from build123d import *

# Parameters (mm, degrees)
BOSS_EXTRUDE1_DEPTH                                  = 300
SKETCH2_R                                            = 30
CUT_EXTRUDE1_DEPTH                                   = 319.198051534
SKETCH3_W                                            = 40
SKETCH3_H                                            = 56
CUT_EXTRUDE2_DEPTH                                   = 10
SKETCH4_W                                            = 40
SKETCH4_H                                            = 49
CUT_EXTRUDE3_DEPTH                                   = 10
FILLET1_R                                            = 3
CSK_FOR_M10_COUNTERSUNK_FLAT_HEAD_SCREW1_D           = 11
CSK_FOR_M10_COUNTERSUNK_FLAT_HEAD_SCREW1_DEPTH       = 20.003
CSK_FOR_M10_COUNTERSUNK_FLAT_HEAD_SCREW1_CSINK_D     = 20
CSK_FOR_M10_COUNTERSUNK_FLAT_HEAD_SCREW1_CSINK_ANGLE = 90
CSK_FOR_M10_COUNTERSUNK_FLAT_HEAD_SCREW1_TIP         = 3.304733405
BOSS_EXTRUDE2_START                                  = -6.35
SKETCH7_R                                            = 30
SKETCH7_R_2                                          = 22.5
BOSS_EXTRUDE2_DEPTH                                  = 6.35
M6X1_0_TAPPED_HOLE1_D                                = 5
M6X1_0_TAPPED_HOLE1_DEPTH                            = 15
M6X1_0_TAPPED_HOLE1_CSINK_D                          = 6.05
M6X1_0_TAPPED_HOLE1_CSINK_ANGLE                      = 90
M6X1_0_TAPPED_HOLE1_TIP                              = 1.502151548


with BuildPart() as part:
    # Sketch1 → Boss-Extrude1 (new body)
    with BuildSketch(Plane.XY):
        Polygon((0, -37.5), (0, 37.5), (75, 37.5), (75, 31.15), (6.35, 31.15), (6.35, -31.15), (75, -31.15), (75, -37.5), align=None)
    extrude(amount=BOSS_EXTRUDE1_DEPTH)

    # Sketch2 → Cut-Extrude1 (cut, through all)
    with BuildSketch(Plane(origin=(0, 37.5, 0), x_dir=(1, 0, 0), z_dir=(0, 1, 0))):
        with Locations(Location((40, -150, 0), (0, 0, 270))):
            Circle(SKETCH2_R)
    extrude(amount=-CUT_EXTRUDE1_DEPTH, mode=Mode.SUBTRACT)

    # Sketch3 → Cut-Extrude2 (cut)
    with BuildSketch(Plane.XZ.offset(37.5)):
        with Locations((40, 63)):
            Rectangle(SKETCH3_W, SKETCH3_H)
    extrude(amount=-CUT_EXTRUDE2_DEPTH, mode=Mode.SUBTRACT)

    # Sketch4 → Cut-Extrude3 (cut)
    with BuildSketch(Plane(origin=(0, 37.5, 0), x_dir=(1, 0, 0), z_dir=(0, 1, 0))):
        with Locations((40, -82.5)):
            Rectangle(SKETCH4_W, SKETCH4_H)
    extrude(amount=-CUT_EXTRUDE3_DEPTH, mode=Mode.SUBTRACT)

    # Fillet1
    fillet1_edges = [part.edges().sort_by_distance(p)[0] for p in [
        (20, -34.325, 91),
        (60, -34.325, 91),
        (60, -34.325, 35),
        (20, -34.325, 35),
        (60, 34.325, 107),
        (20, 34.325, 107),
        (20, 34.325, 58),
        (60, 34.325, 58),
    ]]
    fillet(fillet1_edges, radius=FILLET1_R)

    # CSK for M10 Countersunk Flat Head Screw1
    with Locations(Plane.ZY):
        with Locations((74.704121605, 4.01110333), (72.25, -17.6)):
            CounterSinkHole(CSK_FOR_M10_COUNTERSUNK_FLAT_HEAD_SCREW1_D / 2, CSK_FOR_M10_COUNTERSUNK_FLAT_HEAD_SCREW1_CSINK_D / 2, depth=CSK_FOR_M10_COUNTERSUNK_FLAT_HEAD_SCREW1_DEPTH, counter_sink_angle=CSK_FOR_M10_COUNTERSUNK_FLAT_HEAD_SCREW1_CSINK_ANGLE)
            with Locations((0, 0, -(CSK_FOR_M10_COUNTERSUNK_FLAT_HEAD_SCREW1_DEPTH + CSK_FOR_M10_COUNTERSUNK_FLAT_HEAD_SCREW1_TIP / 2))):  # 118° drill point
                Cone(0, CSK_FOR_M10_COUNTERSUNK_FLAT_HEAD_SCREW1_D / 2, CSK_FOR_M10_COUNTERSUNK_FLAT_HEAD_SCREW1_TIP, mode=Mode.SUBTRACT)

    # Sketch7 → Boss-Extrude2 (add)
    with BuildSketch(Plane.XZ.offset(37.5).offset(BOSS_EXTRUDE2_START)):
        with Locations(Location((40, 150, 0), (0, 0, 90))):
            Circle(SKETCH7_R)
        with Locations(Location((40, 150, 0), (0, 0, 270))):
            Circle(SKETCH7_R_2, mode=Mode.SUBTRACT)
    extrude(amount=BOSS_EXTRUDE2_DEPTH)

    # M6x1.0 Tapped Hole1
    with Locations(Plane(origin=(0, 37.5, 0), x_dir=(1, 0, 0), z_dir=(0, 1, 0))):
        with Locations((66.870057685, -123.129942315), (13.129942315, -123.129942315), (13.129942315, -176.870057685), (66.870057685, -176.870057685)):
            CounterSinkHole(M6X1_0_TAPPED_HOLE1_D / 2, M6X1_0_TAPPED_HOLE1_CSINK_D / 2, depth=M6X1_0_TAPPED_HOLE1_DEPTH, counter_sink_angle=M6X1_0_TAPPED_HOLE1_CSINK_ANGLE)
            with Locations((0, 0, -(M6X1_0_TAPPED_HOLE1_DEPTH + M6X1_0_TAPPED_HOLE1_TIP / 2))):  # 118° drill point
                Cone(0, M6X1_0_TAPPED_HOLE1_D / 2, M6X1_0_TAPPED_HOLE1_TIP, mode=Mode.SUBTRACT)


solid = part.part
Verification items for the finished model (mm, model axes). A direction names the side the tool comes from. Coordinates: 2 decimals unless noted, no trailing zeros. Write each loop counter-clockwise with the first axis right and the second up, starting at its lowest first coordinate (ties: lowest second). Pieces come first, ordered by that corner, then holes. Notation, with made-up numbers: M -33.5,-25.75 L 6.5,-25.75 A23 cw 6.5,2.25 Z; hole C 33,73.25 d5. An arc over 180 degrees is marked long. Use CSV: the item, a comma, the result in double quotes.
Q1. Section check C-C, the plane x = 40. Enter the section's corners in (y, z), and give its area (3 significant figures).
Computed values:
outline,"M -37.5,0 L -31.15,0 L -31.15,35 L -37.5,35 Z; M -37.5,91 L -31.15,91 L -31.15,127.5 L -37.5,127.5 Z; M -37.5,172.5 L -31.15,172.5 L -31.15,300 L -37.5,300 Z; M 31.15,0 L 37.5,0 L 37.5,58 L 31.15,58 Z; M 31.15,107 L 37.5,107 L 37.5,120 L 31.15,120 Z; M 31.15,180 L 37.5,180 L 37.5,300 L 31.15,300 Z"
area,"2,480 mm²"
Q2. Thickness scan on line 1 along Y through (x, z) = (24, 120); line 2 along X through (y, z) = (33, 150); line 3 along X through (y, z) = (24, 254.5). Record the ranges inside material, lowest first. Write a range as [from, to].
Computed values:
line 1,"[-37.5, -31.15], [31.15, 37.5]"
line 2,"[0, 10], [70, 75]"
line 3,"[0, 6.35]"
Q3. Mould release check, pull along Z, two halves, no side actions. Record for faces 6 (the cylindrical face through (12, 34, 179.1)), 7 (the flat face through (37, 37.5, 181)), 8 (the flat face through (4, -5, 0)): pulls with the +Z half, pulls with the -Z half, needs draft (parallel to the pull), parting line crosses it, or undercut.
Computed values:
face 6,"undercut"
face 7,"needs draft"
face 8,"pulls with the -Z half"
Q4. Go/stop test with flat-tipped pins: P1, Ø4, axis at y = 1.5, z = 189.5, coming from the +X side; P2, Ø3, axis at x = 50.5, z = 170, coming from the +Y side. Record where each tip stops, or that it passes through.
Computed values:
P1,"x = 6.35"
P2,"y = -31.15"
Q5. Set-up check for faces 1 (the flat face through (20, -34, 63)), 2 (the flat face through (41, 31.15, 181)), 3 (the cylindrical face through (31.382, -34.281, 129.216)), 4 (the cylindrical face through (13.46, 34.02, 120.65)), 5 (the flat face through (0, -1, 148)): record each of +Z, -Z, +X, -X, +Y, -Y from which the full face is reachable in a straight line by a thin tool's end or side.
Computed values:
face 1,"-Y"
face 2,"+Z, -Z, +X"
face 3,"+Y, -Y"
face 4,"+Y"
face 5,"+Z, -Z, -X, +Y, -Y"
Q6. Section check A-A, the plane z = 150. Enter the section's corners in (x, y), and give its area (3 significant figures).
Computed values:
outline,"M 0,-37.5 L 17.5,-37.5 L 17.5,-31.15 L 6.35,-31.15 L 6.35,31.15 L 10,31.15 L 10,37.5 L 0,37.5 Z; M 62.5,-37.5 L 75,-37.5 L 75,-31.15 L 62.5,-31.15 Z; M 70,31.15 L 75,31.15 L 75,37.5 L 70,37.5 Z"
area,"681 mm²"
Q7. Section check D-D, the plane z = 207. Enter the section's corners in (x, y).
Computed values:
outline,"M 0,-37.5 L 75,-37.5 L 75,-31.15 L 6.35,-31.15 L 6.35,31.15 L 75,31.15 L 75,37.5 L 0,37.5 Z"
Q8. Section check B-B, the plane y = -17.6. Enter the section's corners in (x, z), and give its area (3 significant figures).
Computed values:
outline,"M 0,0 L 6.35,0 L 6.35,66.75 L 4.5,66.75 L 0,62.25 Z; M 0,82.25 L 4.5,77.75 L 6.35,77.75 L 6.35,300 L 0,300 Z"
area,"1,810 mm²"
